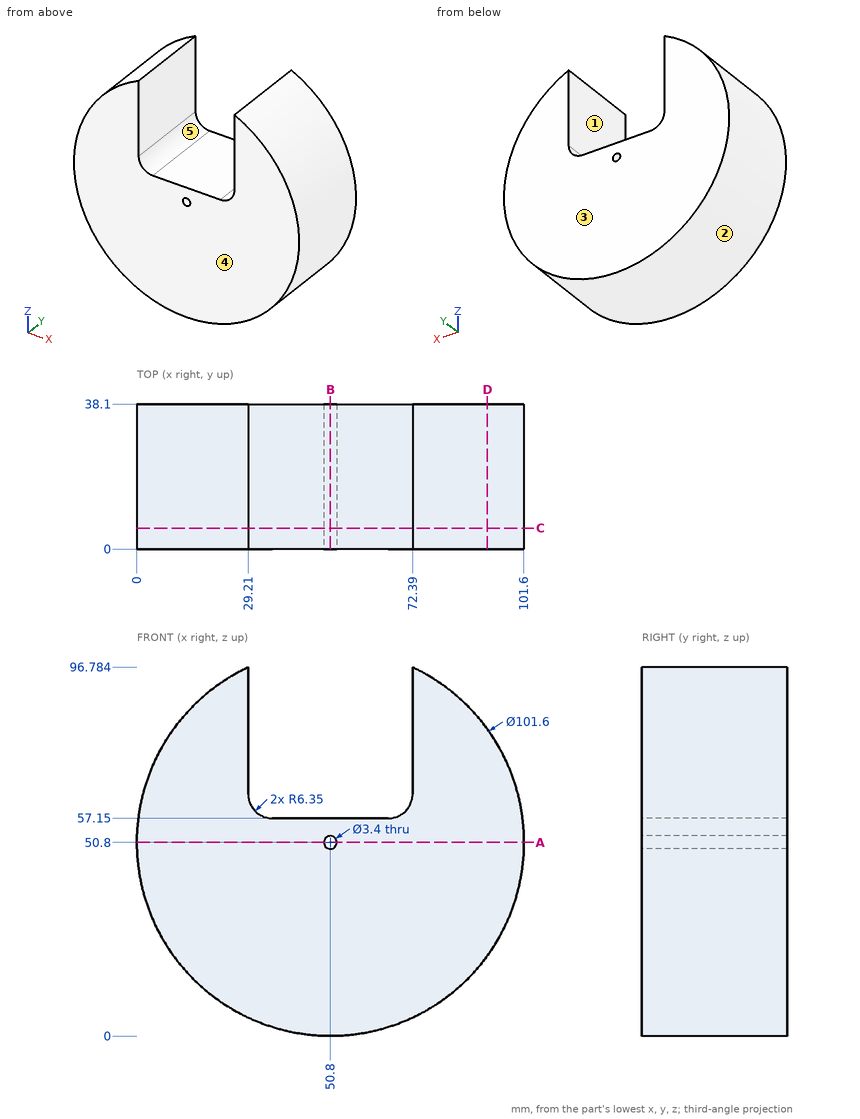
Job drawing, mm, ordinate dimensions from the low corner. One solid piece. A direction names the side the tool comes from. Coordinates: 2 decimals unless noted, no trailing zeros. Write each loop counter-clockwise with the first axis right and the second up, starting at its lowest first coordinate (ties: lowest second). Pieces come first, ordered by that corner, then holes. Notation, with made-up numbers: (62.25, -20.75) - (116.25, -20.75) arc R21 ccw to (116.25, 12.25) - close; hole circle Ø6 at (9.5, 41.5). An arc over 180 degrees is marked (long way). Use a Markdown table: item, result. Add a question column.
Item 1: 3-axis set-ups, long thin cutter, end or side, ignore diameter. For the marked faces 4 and 5: which of +Z, -Z, +X, -X, +Y, -Y reach the whole face in a straight line?
Item 2: Drill centre lines: L1, parallel to Z at x = 50.8, y = 9.5; L2, parallel to X at y = 23.5, z = 50.8; L3, parallel to X at y = 24, z = 50. Where is each one in solid material? Low to high. Write a range as from..to.
Item 3: Flat gauge pins, fed straight in: pin 1 (8 mm diameter, centred on y = 15.5, z = 12, fed in from -X); pin 2 (8 mm diameter, centred on x = 65, y = 17, fed in from +Z); pin 3 (15 mm diameter, centred on x = 57, y = 14, fed in from +Z). Where does each tip first touch, or does it go through?
Item 4: Mould opens along X. For the marked faces 1, 2 and 3 say: pulls with the +X half, pulls with the -X half, needs draft (parallel to the pull), parting line crosses it, or undercut.
Item 5: Band-saw the part on B-B, the plane x = 50.8. Give the cut face in (y, z), and give its area (3 significant figures).
Item 6: Band-saw the part on A-A, the plane z = 50.8. Give the cut face in (x, y), and give its area (3 significant figures).
Item 7: Band-saw the part on D-D, the plane x = 92. Give the cut face in (y, z).
Item 8: Band-saw the part on C-C, the plane y = 5.5. Give the cut face in (x, z), and give its area (3 significant figures).
Numbers:
| question | item | result |
|---|---|---|
| 1 | face 4 | +Z, -Z, +X, -X, -Y |
| 1 | face 5 | +Z, +Y, -Y |
| 2 | L1 | 0..49.1, 52.5..57.15 |
| 2 | L2 | 0..49.1, 52.5..101.6 |
| 2 | L3 | 0.01..49.3, 52.3..101.59 |
| 3 | pin 1 | x = 13.79 |
| 3 | pin 2 | z = 57.88 |
| 3 | pin 3 | z = 57.15 |
| 4 | face 1 | undercut |
| 4 | face 2 | parting line crosses it |
| 4 | face 3 | needs draft |
| 5 | outline | (0, 0) - (38.1, 0) - (38.1, 49.1) - (0, 49.1) - close; (0, 52.5) - (38.1, 52.5) - (38.1, 57.15) - (0, 57.15) - close |
| 5 | area | 2,050 mm2 |
| 6 | outline | (0, 0) - (49.1, 0) - (49.1, 38.1) - (0, 38.1) - close; (52.5, 0) - (101.6, 0) - (101.6, 38.1) - (52.5, 38.1) - close |
| 6 | area | 3,740 mm2 |
| 7 | outline | (0, 21.08) - (38.1, 21.08) - (38.1, 80.52) - (0, 80.52) - close |
| 8 | outline | (29.21, 63.5) - (29.21, 96.78) arc R50.8 ccw (long way) to (72.39, 96.78) - (72.39, 63.5) arc R6.35 cw to (66.04, 57.15) - (35.56, 57.15) arc R6.35 cw to start; hole circle Ø3.4 at (50.8, 50.8) |
| 8 | area | 6,260 mm2 |
